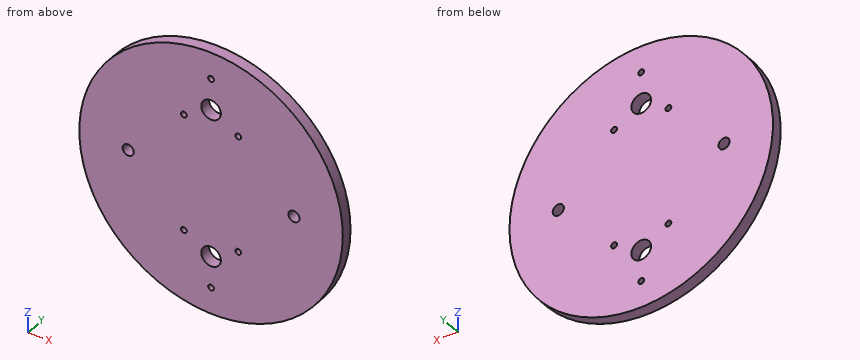
from build123d import *

# Parameters (mm, degrees)
SKETCH1_R                  = 74.676
BOSS_EXTRUDE1_DEPTH        = 6.35
SKETCH2_R                  = 1.651
SKETCH2_R_2                = 5.5626
CO2EJEC_FLANGE_HOLES_DEPTH = 6.35
SKETCH3_R                  = 3.175
F_1_4_HOLES_DEPTH          = 6.35


with BuildPart() as part:
    # Sketch1 → Boss-Extrude1 (new body)
    with BuildSketch(Plane(origin=(0, 0, 0), x_dir=(1, 0, 0), z_dir=(0, 1, 0))):
        Circle(SKETCH1_R)
    extrude(amount=BOSS_EXTRUDE1_DEPTH)

    # Sketch2 → CO2Ejec_Flange_Holes (cut)
    with BuildSketch(Plane(origin=(0, 6.35, 0), x_dir=(1, 0, 0), z_dir=(0, 1, 0))):
        with Locations((15.397931679, 33.02)):
            Circle(SKETCH2_R)
        with Locations((0, 41.91)):
            Circle(SKETCH2_R_2)
        with Locations((0, 59.69)):
            Circle(SKETCH2_R)
        with Locations((-15.397931679, 33.02)):
            Circle(SKETCH2_R)
        with Locations((0, -59.69)):
            Circle(SKETCH2_R)
        with Locations((-15.397931679, -33.02)):
            Circle(SKETCH2_R)
        with Locations((0, -41.91)):
            Circle(SKETCH2_R_2)
        with Locations((15.397931679, -33.02)):
            Circle(SKETCH2_R)
    extrude(amount=-CO2EJEC_FLANGE_HOLES_DEPTH, mode=Mode.SUBTRACT)

    # Sketch3 → 1/4 Holes (cut)
    with BuildSketch(Plane(origin=(0, 6.35, 0), x_dir=(1, 0, 0), z_dir=(0, 1, 0))):
        with Locations((-46.99, 0)):
            Circle(SKETCH3_R)
        with Locations((46.99, 0)):
            Circle(SKETCH3_R)
    extrude(amount=-F_1_4_HOLES_DEPTH, mode=Mode.SUBTRACT)


solid = part.part
Design review of the part built by this model. Coordinates are the model's own, in mm. Coordinates: 2 decimals unless noted, no trailing zeros. Loops run counter-clockwise (first coordinate to the right, second up) from the corner with the lowest first, then second, coordinate; pieces in that order, holes last. Notation, with made-up numbers: (16, -26.5) - (26, -26.5) arc R17 cw to (26, -3.5) - close; hole circle Ø2 at (48.25, -32). An arc over 180 degrees is marked (long way). Use CSV: the item, a comma, the result in double quotes. Start each with the question number.
1. Clearance check with flat-ended pins moving along their axes: pin 1 (2.5 mm diameter, centred on x = -15.4, z = 33.02, fed in from +Y); pin 2 (1 mm diameter, centred on x = 37, y = 5.5, fed in from +Z). State where each tip first meets the part, or that it passes through.
2. Add section C-C on x = -3.5. Give the boundary of the cut face in (y, z).
3. To check wall thickness, follow probe 1 along Z at (x, y) = (0, 3); probe 2 along X at (y, z) = (5.25, 33.02); probe 3 along X at (y, z) = (6, -0.5). State the ranges of each line that lie inside material, in increasing order.
4. Add section B-B on y = 3.5. Count the separate pieces of the cut face and the enclosed holes in it, plus the area to 3 significant figures.
5. Add section A-A on z = 0. Give the boundary of the cut face in (x, y) (3 decimals).
6. Add section D-D on x = -46.99. Give the boundary of the cut face in (y, z) (3 decimals), plus the area to 3 significant figures.
Resolved:
1,pin 1,"through"
1,pin 2,"z = 65.15"
2,outline,"(0, -74.59) - (6.35, -74.59) - (6.35, -46.23) - (0, -46.23) - close; (0, -37.59) - (6.35, -37.59) - (6.35, 37.59) - (0, 37.59) - close; (0, 46.23) - (6.35, 46.23) - (6.35, 74.59) - (0, 74.59) - close"
3,probe 1,"-74.68 to -61.34, -58.04 to -47.47, -36.35 to 36.35, 47.47 to 58.04, 61.34 to 74.68"
3,probe 2,"-66.98 to -17.05, -13.75 to 13.75, 17.05 to 66.98"
3,probe 3,"-74.67 to -50.13, -43.85 to 43.85, 50.13 to 74.67"
4,separate pieces,"1"
4,enclosed holes,"10"
4,area,"17,200 mm2"
5,outline,"(-74.676, 0) - (-50.165, 0) - (-50.165, 6.35) - (-74.676, 6.35) - close; (-43.815, 0) - (43.815, 0) - (43.815, 6.35) - (-43.815, 6.35) - close; (50.165, 0) - (74.676, 0) - (74.676, 6.35) - (50.165, 6.35) - close"
6,outline,"(0, -58.038) - (6.35, -58.038) - (6.35, -3.175) - (0, -3.175) - close; (0, 3.175) - (6.35, 3.175) - (6.35, 58.038) - (0, 58.038) - close"
6,area,"697 mm2"
